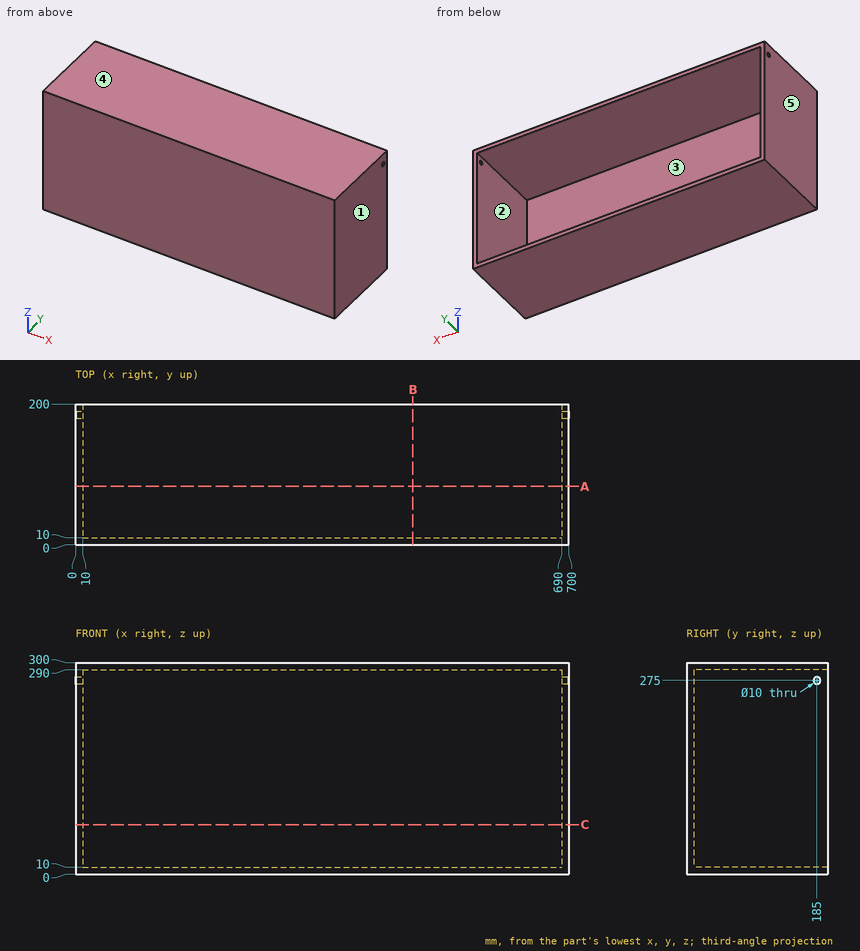
The figure shows three views and two pictorial views of one solid part (mm, origin at its lowest corner). Answer the questions. A direction names the side the tool comes from. Round coordinates to 2 decimals unless told otherwise and drop trailing zeros. Order: outer loops, then holes, each group sorted by start corner. A loop starts at its lowest first (then second) coordinate and runs counter-clockwise, first axis right, second up. Notation, with made-up numbers: (88.25, 77.5) -> (146.25, 77.5) arc R16 cw to (146.25, 88.5) -> close; hole circle Ø9 at (-39, 60). An arc over 180 degrees is marked (long way). Put each result on its own line as item: value.
Q1. This flat-tipped pin is pushed along its axis until it touches: P1, Ø1.5, axis at x = 440, z = 49, coming from the +Y side. Where does it stop, or does it pass through?
Results list:
P1: y = 10
Q2. Section B-B, the plane x = 479 is taken. Write down the section's boundary in (y, z).
Results list:
outline: (0, 0) -> (200, 0) -> (200, 10) -> (10, 10) -> (10, 290) -> (200, 290) -> (200, 300) -> (0, 300) -> close
Q3. Section A-A, the plane y = 83 is taken. Write down the section's boundary in (x, z), and give its area (3 significant figures).
Results list:
outline: (0, 0) -> (700, 0) -> (700, 300) -> (0, 300) -> close; hole (10, 10) -> (690, 10) -> (690, 290) -> (10, 290) -> close
area: 19,600 mm^2
Q4. Which of the six approach directions +Z, -Z, +X, -X, +Y, -Y give full straight-line access (tool end or side, diameter ignored) to the marked faces 1 and 2?
Results list:
face 1: +Z, -Z, +X, +Y, -Y
face 2: +Y
Q5. Consider line 1 along X through (y, z) = (43.5, 29.5); line 2 along Z through (x, y) = (354, 11.5); line 3 along Y through (x, z) = (4.25, 275). Determine where each line is inside the solid, lowest interval first.
Results list:
line 1: 0 to 10, 690 to 700
line 2: 0 to 10, 290 to 300
line 3: 0 to 180, 190 to 200
Q6. Section C-C, the plane z = 70.5 is taken. Write down the section's boundary in (x, y).
Results list:
outline: (0, 0) -> (700, 0) -> (700, 200) -> (690, 200) -> (690, 10) -> (10, 10) -> (10, 200) -> (0, 200) -> close
Q7. Determine the mould class of the marked faces 3, 4 and 5 for opening direction X: pulls with the +X half, pulls with the -X half, needs draft (parallel to the pull), parting line crosses it, or undercut.
Results list:
face 3: undercut
face 4: needs draft
face 5: pulls with the -X half
